```python
from build123d import *

# Parameters (mm, degrees)
F1_DEPTH = 100
F3_DEPTH = 50


with BuildPart() as f1:
    # F0 (on Front) → F1 (new body)
    with BuildSketch(Plane.XZ):
        Polygon((-50, 100), (-100, 100), (-100, 0), (0, 0), (0, 50), align=None)
    extrude(amount=F1_DEPTH)

    # F2 (on face) → F3 (cut)
    with BuildSketch(Plane.XZ.offset(100)):
        Polygon((0, 50), (-50, 100), (-50, 50), align=None)
    extrude(amount=-F3_DEPTH, mode=Mode.SUBTRACT)


solid = f1.part
```
Work out the finished part from the listing and answer in its coordinate system (mm). A direction names the side the tool comes from. Coordinates: 2 decimals unless noted, no trailing zeros. Loops run counter-clockwise (first coordinate to the right, second up) from the corner with the lowest first, then second, coordinate; pieces in that order, holes last. Notation, with made-up numbers: (4, 50) - (54, 50) arc R24 cw to (54, 74) - close; hole circle Ø2 at (4.25, -35.75). An arc over 180 degrees is marked (long way). Use a Markdown table: item, result.
Item 1: Consider probe 1 along X at (y, z) = (-55.5, 82.5); probe 2 along Y at (x, z) = (-26, 75); probe 3 along Z at (x, y) = (-12, -62). Determine where each line is inside the solid, lowest interval first. Write a range as from..to.
Evaluation:
| item | result |
|---|---|
| probe 1 | x = -100..-50 |
| probe 2 | y = -50..0 |
| probe 3 | z = 0..50 |
Item 2: Find section A-A, the plane y = -39. Determine the outline of the cut face in (x, z), and give its area (3 significant figures).
Evaluation:
| item | result |
|---|---|
| outline | (-100, 0) - (0, 0) - (0, 50) - (-50, 100) - (-100, 100) - close |
| area | 8,750 mm2 |
Item 3: Find section B-B, the plane z = 87. Determine the outline of the cut face in (x, y).
Evaluation:
| item | result |
|---|---|
| outline | (-100, -100) - (-50, -100) - (-50, -50) - (-37, -50) - (-37, 0) - (-100, 0) - close |
Item 4: Find section C-C, the plane x = -37.5. Determine the outline of the cut face in (y, z), and give its area (4 significant figures).
Evaluation:
| item | result |
|---|---|
| outline | (-100, 0) - (0, 0) - (0, 87.5) - (-50, 87.5) - (-50, 50) - (-100, 50) - close |
| area | 6,875 mm2 |
Item 5: For faces 1 (the flat face through (-75, -49, 100)), 2 (the flat face through (-50, -75, 75)), determine the directions among +Z, -Z, +X, -X, +Y, -Y from which every point of the face is accessible in a straight line to the end or side of a thin tool.
Evaluation:
| item | result |
|---|---|
| face 1 | +Z, +X, -X, +Y, -Y |
| face 2 | +Z, +X, -Y |
Item 6: Given pin 1 Ø15 at (x, y) = (-36.5, -77.5) entering from +Z; pin 2 Ø5 at (x, z) = (-43.5, 76) entering from -Y; pin 3 Ø5 at (x, y) = (-45.5, -43) entering from +Z; pin 4 Ø1 at (x, z) = (-60, 64.5) entering from +Y, each flat-ended and moving along its own axis, determine where each tip first touches the part or whether it passes through.
Evaluation:
| item | result |
|---|---|
| pin 1 | stops at z = 50 |
| pin 2 | stops at y = -50 |
| pin 3 | stops at z = 98 |
| pin 4 | stops at y = 0 |
